```python
from build123d import *

# Parameters (mm, degrees)
BOSS_EXTRUDE1_DEPTH = 2
SWEEP2_PROFILE_R    = 5
INTERSECT1_START    = -2
INTERSECT1_DEPTH    = 4


# Read off the part's stored shape, not the designer's step: Intersect1
with BuildPart() as part:
    # Sketch1 → Boss-Extrude1 (new, symmetric)
    with BuildSketch(Plane(origin=(0, 0, 0), x_dir=(1, 0, 0), z_dir=(0, 1, 0))):
        with BuildLine():
            Line((-52.048116563, 47.218434745), (24.754223647, 47.218434745))
            ThreePointArc((24.754223647, 47.218434745), (31.825291459, 44.289502557), (34.754223647, 37.218434745))
            Line((34.754223647, 37.218434745), (34.754223647, -55.414363356))
            ThreePointArc((34.754223647, -55.414363356), (31.825291459, -62.485431168), (24.754223647, -65.414363356))
            Line((24.754223647, -65.414363356), (-52.048116563, -65.414363356))
            ThreePointArc((-52.048116563, -65.414363356), (-59.119184375, -62.485431168), (-62.048116563, -55.414363356))
            Line((-62.048116563, -55.414363356), (-62.048116563, 37.218434745))
            ThreePointArc((-62.048116563, 37.218434745), (-59.119184375, 44.289502557), (-52.048116563, 47.218434745))
        make_face()
    extrude(amount=BOSS_EXTRUDE1_DEPTH, both=True)


with BuildPart() as body_2:
    # Sweep2: sweep along a path in Sketch1<3>
    with BuildLine(Plane(origin=(0, 0, 0), x_dir=(1, 0, 0), z_dir=(0, 1, 0))) as sweep2_path:
        Line((-52.048116563, 47.218434745), (24.754223647, 47.218434745))
        ThreePointArc((24.754223647, 47.218434745), (31.825291459, 44.289502557), (34.754223647, 37.218434745))
        Line((34.754223647, 37.218434745), (34.754223647, -55.414363356))
        ThreePointArc((34.754223647, -55.414363356), (31.825291459, -62.485431168), (24.754223647, -65.414363356))
        Line((24.754223647, -65.414363356), (-52.048116563, -65.414363356))
        ThreePointArc((-52.048116563, -65.414363356), (-59.119184375, -62.485431168), (-62.048116563, -55.414363356))
        Line((-62.048116563, -55.414363356), (-62.048116563, 37.218434745))
        ThreePointArc((-62.048116563, 37.218434745), (-59.119184375, 44.289502557), (-52.048116563, 47.218434745))
    # Sweep2 profile (on start of the path) → Sweep2 (sweep)
    with BuildSketch(Plane(origin=(-52.048116563, 0, -47.218434745), x_dir=(0, 0, 1), z_dir=(1, 0, 0))):
        Circle(SWEEP2_PROFILE_R)
    sweep(path=sweep2_path.line)


with BuildPart() as intersect1_tool:
    # Intersect1 outline → Intersect1 (new body)
    with BuildSketch(Plane(origin=(0, 0, 0), x_dir=(1, 0, 0), z_dir=(0, 1, 0)).offset(INTERSECT1_START)):
        with BuildLine():
            ThreePointArc((-52.048116563, 47.218434745), (-59.119184375, 44.289502557), (-62.048116563, 37.218434745))
            Line((-62.048116563, 37.218434745), (-62.048116563, -55.414363356))
            ThreePointArc((-62.048116563, -55.414363356), (-59.119184375, -62.485431168), (-52.048116563, -65.414363356))
            Line((-52.048116563, -65.414363356), (24.754223647, -65.414363356))
            ThreePointArc((24.754223647, -65.414363356), (31.825291459, -62.485431168), (34.754223647, -55.414363356))
            Line((34.754223647, -55.414363356), (34.754223647, 37.218434745))
            ThreePointArc((34.754223647, 37.218434745), (31.825291459, 44.289502557), (24.754223647, 47.218434745))
            Line((24.754223647, 47.218434745), (-52.048116563, 47.218434745))
        make_face()
    extrude(amount=INTERSECT1_DEPTH)


with BuildPart() as part_1:
    add(part.part)

    # Intersect1: cut by intersect1_tool
    add(intersect1_tool.part, mode=Mode.SUBTRACT)


with BuildPart() as body_2_1:
    add(body_2.part)

    # Intersect1: cut by intersect1_tool
    add(intersect1_tool.part, mode=Mode.SUBTRACT)


solid = body_2_1.part
```
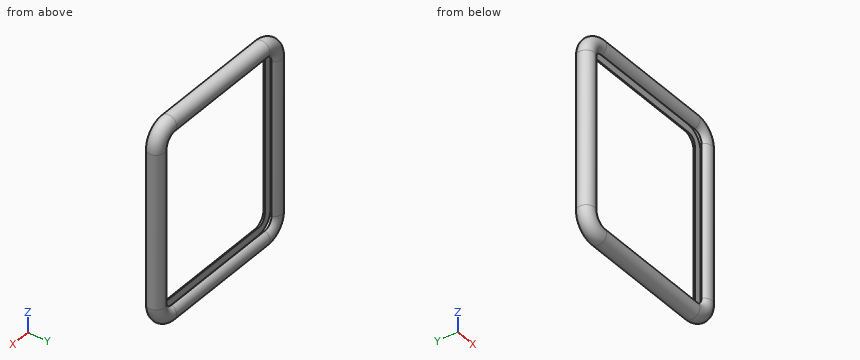
Check sheet for the modelled part. Datum: model origin and axes. Units: mm. Give positions to 0.01 mm unless a question says otherwise; leave off trailing zeros. Loops run counter-clockwise (first coordinate to the right, second up) from the corner with the lowest first, then second, coordinate; pieces in that order, holes last. Notation, with made-up numbers: (-12, 11.25) - (42, 11.25) arc R21 ccw to (42, 42.25) - close; hole circle Ø6 at (-20, 85.5). An arc over 180 degrees is marked (long way). One line per question, with ' | ' between items. Start each with the question number.
1. Gauge pin test, flat ends, axial feed: pin 1 Ø2 at (y, z) = (-3, -10.5) entering from +X; pin 2 Ø1.5 at (y, z) = (-1, -19) entering from -X; pin 3 Ø3 at (x, y) = (-8.5, 3) entering from +Z. Record the tip position at first contact, or that the pin passes through.
2. Cross-section at A-A, the plane z = 2. Enter the section's corners in (x, y).
3. Cross-section at C-C, the plane y = 3.5. Enter the section's corners in (x, z), plus the area to 3 significant figures.
4. Material ranges on line 1 along Z through (x, y) = (15.5, 0.25); line 2 along X through (y, z) = (0, 17); line 3 along Y through (x, z) = (-45, 61), recorded low to high. Write a range as [from, to].
5. Cross-section at B-B, the plane x = -17. Enter the section's corners in (y, z), plus the area to 3 significant figures.
Check result:
1) pin 1: stops at x = 39.34 | pin 2: stops at x = -67.04 | pin 3: stops at z = 70.18
2) outline: (-62.05, -2) - (-62.05, 2) - (-57.47, 2) arc R5 ccw (long way) to (-57.47, -2) - close; (30.17, -2) arc R5 ccw (long way) to (30.17, 2) - (34.75, 2) - (34.75, -2) - close
3) outline: (-65.62, -37.22) arc R13.57 ccw to (-52.05, -50.79) - (24.75, -50.79) arc R13.57 ccw to (38.32, -37.22) - (38.32, 55.41) arc R13.57 ccw to (24.75, 68.99) - (-52.05, 68.99) arc R13.57 ccw to (-65.62, 55.41) - close; hole (-58.48, -37.22) arc R6.43 ccw to (-52.05, -43.65) - (24.75, -43.65) arc R6.43 ccw to (31.18, -37.22) - (31.18, 55.41) arc R6.43 ccw to (24.75, 61.84) - (-52.05, 61.84) arc R6.43 ccw to (-58.48, 55.41) - close | area: 2,870 mm2
4) line 1: z = [-52.21, -47.22], [65.41, 70.41] | line 2: x = [-67.05, -62.05], [34.75, 39.75] | line 3: y = [-2.35, -2], [2, 2.35]
5) outline: (-2, -47.22) - (-2, -42.64) arc R5 ccw (long way) to (2, -42.64) - (2, -47.22) - close; (-2, 60.83) - (-2, 65.41) - (2, 65.41) - (2, 60.83) arc R5 ccw (long way) to start | area: 118 mm2
